Part model, mm, in its own coordinate system. Face numbers are marked on the shaded views. A direction names the side the tool comes from. Give positions to 0.01 mm unless a question says otherwise; leave off trailing zeros. Write each loop counter-clockwise with the first axis right and the second up, starting at its lowest first coordinate (ties: lowest second). Pieces come first, ordered by that corner, then holes. Notation, with made-up numbers: M -34.75,47.5 L -18.75,47.5 A18 cw -18.75,71.5 Z; hole C -19,87 d4. An arc over 180 degrees is marked long. Use a Markdown table: item, result. Add a question column.
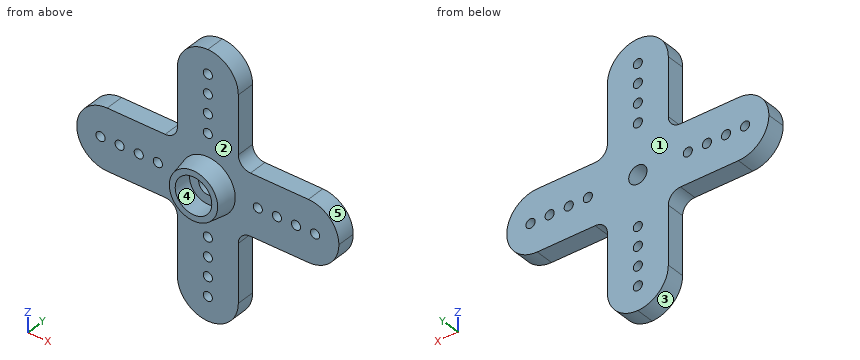
from build123d import *

# Parameters (mm, degrees)
BOSS_EXTRUDE1_DEPTH = 3
FILLET1_R           = 2
FILLET2_R           = 5
SKETCH2_R           = 4.5
BOSS_EXTRUDE2_DEPTH = 3
DRAFT1_ANGLE        = 10
SKETCH3_R           = 3
CUT_EXTRUDE1_DEPTH  = 3
SKETCH4_R           = 1.5
CUT_EXTRUDE2_DEPTH  = 31.553232235
SKETCH5_R           = 0.75
CUT_EXTRUDE3_DEPTH  = 31.991934435
CIRPATTERN1_COUNT   = 4


with BuildPart() as part:
    # Sketch1 → Boss-Extrude1 (new body)
    with BuildSketch(Plane(origin=(0, 0, 0), x_dir=(1, 0, 0), z_dir=(0, 1, 0))):
        Polygon((-5, 5), (-5, 21.5), (5, 21.5), (5, 5), (21.5, 5), (21.5, -5), (5, -5), (5, -21.5), (-5, -21.5), (-5, -5), (-21.5, -5), (-21.5, 5), align=None)
    extrude(amount=BOSS_EXTRUDE1_DEPTH)

    # Fillet1
    fillet1_edges = [part.edges().sort_by_distance(p)[0] for p in [
        (-5, 1.5, -5),
        (5, 1.5, -5),
        (5, 1.5, 5),
        (-5, 1.5, 5),
    ]]
    fillet(fillet1_edges, radius=FILLET1_R)

    # Fillet2
    fillet2_edges = [part.edges().sort_by_distance(p)[0] for p in [
        (-21.5, 1.5, -5),
        (-5, 1.5, -21.5),
        (-21.5, 1.5, 5),
        (5, 1.5, -21.5),
        (21.5, 1.5, -5),
        (21.5, 1.5, 5),
        (5, 1.5, 21.5),
        (-5, 1.5, 21.5),
    ]]
    fillet(fillet2_edges, radius=FILLET2_R - 0.0001)  # a hair under: the kernel refuses the full size

    # Sketch2 → Boss-Extrude2 (add)
    with BuildSketch(Plane.XZ):
        with Locations(Location((0, 0, 0), (0, 0, 90))):
            Circle(SKETCH2_R)
    extrude(amount=BOSS_EXTRUDE2_DEPTH)

    # Draft1
    draft1_faces = [part.faces().sort_by_distance(p)[0] for p in [
        (0, -1.5, -4.5),
    ]]
    draft(draft1_faces, Plane(origin=(0, 0, 0), x_dir=(0, 0, -1), z_dir=(0, -1, 0)), DRAFT1_ANGLE)

    # Sketch3 → Cut-Extrude1 (cut)
    with BuildSketch(Plane.XZ.offset(3)):
        with Locations(Location((0, 0, 0), (0, 0, 270))):
            Circle(SKETCH3_R)
    extrude(amount=-CUT_EXTRUDE1_DEPTH, mode=Mode.SUBTRACT)

    # Sketch4 → Cut-Extrude2 (cut, through all)
    with BuildSketch(Plane.XZ):
        with Locations(Location((0, 0, 0), (0, 0, 270))):
            Circle(SKETCH4_R)
    extrude(amount=-CUT_EXTRUDE2_DEPTH, mode=Mode.SUBTRACT)

    # Sketch5 → Cut-Extrude3 (cut, through all)
    with BuildSketch(Plane(origin=(0, 3, 0), x_dir=(1, 0, 0), z_dir=(0, 1, 0))):
        with Locations(Location((0, 17.6, 0), (0, 0, 270))):
            Circle(SKETCH5_R)
        with Locations(Location((0, 14.466666667, 0), (0, 0, 270))):
            Circle(SKETCH5_R)
        with Locations(Location((0, 11.333333333, 0), (0, 0, 270))):
            Circle(SKETCH5_R)
        with Locations(Location((0, 8.2, 0), (0, 0, 270))):
            Circle(SKETCH5_R)
    cut_extrude3 = extrude(amount=-CUT_EXTRUDE3_DEPTH, mode=Mode.SUBTRACT)

    # CirPattern1: Cut-Extrude3 ×4 about axis
    cirpattern1_axis = Axis((0, 0, 0), (0, 1, 0))
    for i in range(1, CIRPATTERN1_COUNT):
        add(cut_extrude3.rotate(cirpattern1_axis, i * 360 / CIRPATTERN1_COUNT), mode=Mode.SUBTRACT)


solid = part.part
1. Cut at D-D (z = 16). Write the cut outline in (x, y), then the cut area to 3 significant figures.
2. Mould opens along X. For the marked faces 3, 4 and 5 say: released by +X, released by -X, zero draft, split by the parting line, or undercut.
3. Cut at A-A (x = -8.2). Write the cut outline in (y, z), then the cut area to 3 significant figures.
4. Cut at C-C (y = 2.15). Give the number of separate pieces and of enclosed holes in the cut face, then the cut area to 3 significant figures.
5. Flat gauge pins, fed straight in: pin 1 (2 mm diameter, centred on x = 17.6, z = 0, fed in from -Y); pin 2 (2 mm diameter, centred on y = 1.5, z = 1.5, fed in from +X); pin 3 (2 mm diameter, centred on x = 12.5, y = 1, fed in from +Z). Where does each tip first touch, or does it go through?
6. Drill centre lines: probe 1 along X at (y, z) = (1.95, -8.2); probe 2 along X at (y, z) = (0.2, -10); probe 3 along X at (y, z) = (0.25, 12). Where is each one in solid material? Low to high. Write a range as [from, to].
7. Cut at B-B (z = -17.6). Write the cut outline in (x, y), then the cut area to 3 significant figures.
8. Tool access for the marked faces 1 and 2: list every direction of +Z, -Z, +X, -X, +Y, -Y with a clear straight run to the whole face (end or side of a thin tool).
A:
| question | item | result |
|---|---|---|
| 1 | outline | M -5,0 L 5,0 L 5,3 L -5,3 Z |
| 1 | area | 30.0 mm² |
| 2 | face 3 | released by -X |
| 2 | face 4 | undercut |
| 2 | face 5 | released by +X |
| 3 | outline | M 0,-5 L 3,-5 L 3,-0.75 L 0,-0.75 Z; M 0,0.75 L 3,0.75 L 3,5 L 0,5 Z |
| 3 | area | 25.5 mm² |
| 4 | separate pieces | 1 |
| 4 | enclosed holes | 17 |
| 4 | area | 685 mm² |
| 5 | pin 1 | stops at y = 0 |
| 5 | pin 2 | stops at x = 21.47 |
| 5 | pin 3 | stops at z = 5 |
| 6 | probe 1 | x = [-5, -0.75], [0.75, 5] |
| 6 | probe 2 | x = [-5, 5] |
| 6 | probe 3 | x = [-5, -0.34], [0.34, 5] |
| 7 | outline | M -4.88,0 L -0.75,0 L -0.75,3 L -4.88,3 Z; M 0.75,0 L 4.88,0 L 4.88,3 L 0.75,3 Z |
| 7 | area | 24.8 mm² |
| 8 | face 1 | +Z, -Z, +X, -X, +Y |
| 8 | face 2 | -Y |
